from build123d import *

# Parameters (mm, degrees)
SKETCH_1_W             = 103.5
SKETCH_1_H             = 10.4
BASE_DEPTH             = 7
SKETCH_3_W             = 30
SKETCH_3_H             = 6
FINGER_CONNECTOR_DEPTH = 9
SKETCH_5_W             = 103.5
SKETCH_5_H             = 2.6
GEAR_CONNECTOR_DEPTH   = 9.85
CUT_EXTRUDE_1_DEPTH    = 1.5
SKETCH_20_R            = 1.425
CUT_EXTRUDE_4_DEPTH    = 106.063897224
SKETCH_22_R            = 1.425
CUT_EXTRUDE_5_DEPTH    = 1
SKETCH_27_R            = 1.675
CUT_EXTRUDE_6_DEPTH    = 10
CHAMFER_2_SIZE         = 1.3


with BuildPart() as part:
    # 草图1 → Base (new body)
    with BuildSketch(Plane(origin=(0, 0, 0), x_dir=(1, 0, 0), z_dir=(0, 1, 0))):
        with Locations((51.75, -5.2)):
            Rectangle(SKETCH_1_W, SKETCH_1_H)
    extrude(amount=BASE_DEPTH)

    # 草图3 → Finger_Connector (add)
    with BuildSketch(Plane(origin=(0, 0, 0), x_dir=(-1, 0, 0), z_dir=(0, -1, 0))):
        with Locations((-88.5, -3)):
            Rectangle(SKETCH_3_W, SKETCH_3_H)
    extrude(amount=FINGER_CONNECTOR_DEPTH)

    # 草图5 → Gear Connector (add)
    with BuildSketch(Plane(origin=(0, 7, 0), x_dir=(1, 0, 0), z_dir=(0, 1, 0))):
        with Locations((51.75, -5.2)):
            Rectangle(SKETCH_5_W, SKETCH_5_H)
    extrude(amount=GEAR_CONNECTOR_DEPTH)

    # 草图6 → 切除-拉伸1 (cut)
    with BuildSketch(Plane.ZY):
        Polygon((3.9, 16.85), (3.9, 7), (0, 7), (0, 0), (10.4, 0), (10.4, 7), (6.5, 7), (6.5, 16.85), align=None)
    extrude(amount=-CUT_EXTRUDE_1_DEPTH, mode=Mode.SUBTRACT)

    # 草图20 → 切除-拉伸4 (cut, through all)
    with BuildSketch(Plane.XY.offset(6.5)):
        with Locations((13.5, 13.6)):
            Circle(SKETCH_20_R)
        with Locations((5.5, 13.6)):
            Circle(SKETCH_20_R)
        with Locations((99.5, 13.6)):
            Circle(SKETCH_20_R)
        with Locations((91.5, 13.6)):
            Circle(SKETCH_20_R)
    extrude(amount=-CUT_EXTRUDE_4_DEPTH, mode=Mode.SUBTRACT)

    # 草图22 → 切除-拉伸5 (cut)
    # profile 1 of 4: a face of its own
    with BuildSketch(Plane.XY.offset(6.5)):
        Polygon((92.998593259, 10.998548179), (94.502219993, 13.597093921), (93.003626735, 16.198545743), (90.001406741, 16.201451821), (88.497780007, 13.602906079), (89.996373265, 11.001454257), align=None)
        with Locations((91.5, 13.6)):
            Circle(SKETCH_22_R, mode=Mode.SUBTRACT)
    # profile 2 of 4: a face of its own
    with BuildSketch(Plane.XY.offset(6.5)):
        Polygon((101.010012931, 11.005160066), (102.502203767, 13.610289591), (100.992190836, 16.205129525), (97.989987069, 16.194839934), (96.497796233, 13.589710409), (98.007809164, 10.994870475), align=None)
        with Locations((99.5, 13.6)):
            Circle(SKETCH_22_R, mode=Mode.SUBTRACT)
    # profile 3 of 4: a face of its own
    with BuildSketch(Plane.XY.offset(6.5)):
        Polygon((15.023964186, 11.013329071), (16.502104828, 13.626456235), (14.978140642, 16.213127164), (11.976035814, 16.186670929), (10.497895172, 13.573543765), (12.021859358, 10.986872836), align=None)
        with Locations((13.5, 13.6)):
            Circle(SKETCH_22_R, mode=Mode.SUBTRACT)
    # profile 4 of 4: a face of its own
    with BuildSketch(Plane.XY.offset(6.5)):
        Polygon((6.985197547, 10.99087724), (8.502165366, 13.581657426), (7.016967818, 16.190780186), (4.014802453, 16.20912276), (2.497834634, 13.618342574), (3.983032182, 11.009219814), align=None)
        with Locations((5.5, 13.6)):
            Circle(SKETCH_22_R, mode=Mode.SUBTRACT)
    extrude(amount=-CUT_EXTRUDE_5_DEPTH, mode=Mode.SUBTRACT)

    # 草图27 → 切除-拉伸6 (cut)
    with BuildSketch(Plane.XY.offset(6)):
        with Locations((98.5, -4.5)):
            Circle(SKETCH_27_R)
        with Locations((88.5, -4.5)):
            Circle(SKETCH_27_R)
        with Locations((78.5, -4.5)):
            Circle(SKETCH_27_R)
    extrude(amount=-CUT_EXTRUDE_6_DEPTH, mode=Mode.SUBTRACT)

    # 倒角2
    chamfer_2_edges = [part.edges().sort_by_distance(p)[0] for p in [
        (76.825, -4.5, 6),
        (86.825, -4.5, 6),
        (96.825, -4.5, 6),
    ]]
    chamfer(chamfer_2_edges, length=CHAMFER_2_SIZE)


solid = part.part
Check sheet for the modelled part. Datum: model origin and axes. Units: mm. A direction names the side the tool comes from. Round coordinates to 2 decimals unless told otherwise and drop trailing zeros. Order: outer loops, then holes, each group sorted by start corner. A loop starts at its lowest first (then second) coordinate and runs counter-clockwise, first axis right, second up.
Q1. Cross-section at D-D, the plane y = 9.5. Enter the section's corners in (x, z).
Filled sheet:
outline: (1.5, 3.9) - (103.5, 3.9) - (103.5, 6.5) - (1.5, 6.5) - close
Q2. Draft check along X on faces 5 (the face through (73.5, -4, 3)), 6 (the face through (52, 16.85, 5)), 7 (the face through (103.5, 4, 4)), 8 (the face through (100.86, 14.03, 4.71)). Enter one of: pulls with the +X half, pulls with the -X half, needs draft (parallel to the pull), parting line crosses it, or undercut.
Filled sheet:
face 5: pulls with the -X half
face 6: needs draft
face 7: pulls with the +X half
face 8: undercut
Q3. Cross-section at B-B, the plane z = 2.75. Enter the section's corners in (x, y) (3 decimals), plus the area to 3 significant figures.
Filled sheet:
outline: (1.5, 0) - (73.5, 0) - (73.5, -9) - (103.5, -9) - (103.5, 7) - (1.5, 7) - close; hole circle Ø3.35 at (78.5, -4.5); hole circle Ø3.35 at (88.5, -4.5); hole circle Ø3.35 at (98.5, -4.5)
area: 958 mm2
Q4. Depth check by flat-ended pin: P1, Ø5, axis at x = 67.5, y = 13.5, coming from the +Z side; P2, Ø1.8, axis at y = -4, z = 2.5, coming from the -X side; P3, Ø3.5, axis at x = 91.5, y = 13.6, coming from the +Z side. Enter the tip coordinate at first touch or a pass-through.
Filled sheet:
P1: stops at z = 6.5
P2: stops at x = 73.5
P3: stops at z = 5.5
Q5. Set-up check for faces 1 (the face through (93, 15, 5.5)), 2 (the face through (52, 12, 6.5)), 3 (the face through (52, 12, 3.9)), 4 (the face through (89, -1, 6)): record each of +Z, -Z, +X, -X, +Y, -Y from which the full face is reachable in a straight line by a thin tool's end or side.
Filled sheet:
face 1: +Z
face 2: +Z, +X, -X, +Y
face 3: -Z, +X, -X, +Y
face 4: +Z, +X, -X, -Y
Q6. Scan lines: L1, parallel to Y at x = 78.5, z = 2.45 (3 decimals); L2, parallel to Y at x = 5.5, z = 4.85 (3 decimals); L3, parallel to Y at x = 26.5, z = 5.5. Record each from-to range of solid material in increasing order.
Filled sheet:
L1: y = -9 to -6.175, -2.825 to 7
L2: y = 0 to 12.175, 15.025 to 16.85
L3: y = 0 to 16.85
Q7. Cross-section at C-C, the plane x = 13.5. Enter the section's corners in (y, z) (3 decimals), plus the area to 4 significant figures.
Filled sheet:
outline: (0, 0) - (7, 0) - (7, 3.9) - (12.175, 3.9) - (12.175, 5.5) - (11, 5.5) - (11, 6.5) - (7, 6.5) - (7, 10.4) - (0, 10.4) - close; (15.025, 3.9) - (16.85, 3.9) - (16.85, 6.5) - (16.2, 6.5) - (16.2, 5.5) - (15.025, 5.5) - close
area: 88.65 mm2
Q8. Cross-section at A-A, the plane y = -4.5. Enter the section's corners in (x, z) (3 decimals).
Filled sheet:
outline: (73.5, 0) - (76.825, 0) - (76.825, 4.7) - (75.525, 6) - (73.5, 6) - close; (80.175, 0) - (86.825, 0) - (86.825, 4.7) - (85.525, 6) - (81.475, 6) - (80.175, 4.7) - close; (90.175, 0) - (96.825, 0) - (96.825, 4.7) - (95.525, 6) - (91.475, 6) - (90.175, 4.7) - close; (100.175, 0) - (103.5, 0) - (103.5, 6) - (101.475, 6) - (100.175, 4.7) - close
